```python
from build123d import *

# Parameters (mm, degrees)
BOSS_EXTRUDE1_DEPTH                                = 12.7
F_1_4_20_TAPPED_HOLE1_D                            = 5.1054
F_1_4_20_TAPPED_HOLE1_DEPTH                        = 12.7
F_1_4_20_TAPPED_HOLE2_D                            = 5.1054
F_1_4_20_TAPPED_HOLE2_DEPTH                        = 12.7
LPATTERN1_COUNT                                    = 3
LPATTERN1_PITCH                                    = 12.7
LPATTERN2_COUNT                                    = 3
LPATTERN2_PITCH                                    = 12.7
CSK_FOR_10_FLAT_HEAD_MACHINE_SCREW_100_D           = 5.1054
CSK_FOR_10_FLAT_HEAD_MACHINE_SCREW_100_DEPTH       = 12.7
CSK_FOR_10_FLAT_HEAD_MACHINE_SCREW_100_CSINK_D     = 9.779
CSK_FOR_10_FLAT_HEAD_MACHINE_SCREW_100_CSINK_ANGLE = 100
F_1_8_0_125_DIAMETER_HOLE1_D                       = 3.175
F_1_8_0_125_DIAMETER_HOLE1_DEPTH                   = 12.7
CSK_FOR_10_FLAT_HEAD_MACHINE_SCREW_2_D             = 5.1054
CSK_FOR_10_FLAT_HEAD_MACHINE_SCREW_2_DEPTH         = 12.7
CSK_FOR_10_FLAT_HEAD_MACHINE_SCREW_2_CSINK_D       = 9.779
CSK_FOR_10_FLAT_HEAD_MACHINE_SCREW_2_CSINK_ANGLE   = 100


with BuildPart() as part:
    # Sketch1 → Boss-Extrude1 (new body)
    with BuildSketch(Plane(origin=(0, 0, 0), x_dir=(1, 0, 0), z_dir=(0, 1, 0))):
        Polygon((24.616308072, 0), (53.826308072, 0), (53.826308072, 40.5892), (24.616308072, 40.5892), (24.616308072, 109.3724), (-0.783691928, 109.3724), (-0.783691928, 52.2224), (7.674508072, 52.2224), (8.4582, -11.6332), (-0.783691928, -11.6332), (-0.783691928, -68.7832), (24.616308072, -68.7832), align=None)
    extrude(amount=BOSS_EXTRUDE1_DEPTH)

    # 1/4-20 Tapped Hole1
    with Locations(Plane(origin=(0, 12.7, 0), x_dir=(1, 0, 0), z_dir=(0, 1, 0))):
        with Locations((9.376308072, 99.2124)):
            f_1_4_20_tapped_hole1 = Hole(F_1_4_20_TAPPED_HOLE1_D / 2, depth=F_1_4_20_TAPPED_HOLE1_DEPTH)

    # 1/4-20 Tapped Hole2
    with Locations(Plane(origin=(0, 12.7, 0), x_dir=(1, 0, 0), z_dir=(0, 1, 0))):
        with Locations((9.376308072, -58.6232)):
            f_1_4_20_tapped_hole2 = Hole(F_1_4_20_TAPPED_HOLE2_D / 2, depth=F_1_4_20_TAPPED_HOLE2_DEPTH)

    # LPattern1: 1/4-20 Tapped Hole1 ×3
    with Locations(*[(0, 0, i * LPATTERN1_PITCH) for i in range(1, LPATTERN1_COUNT)]):
        add(f_1_4_20_tapped_hole1, mode=Mode.SUBTRACT)

    # LPattern2: 1/4-20 Tapped Hole2 ×3
    with Locations(*[(0, 0, -i * LPATTERN2_PITCH) for i in range(1, LPATTERN2_COUNT)]):
        add(f_1_4_20_tapped_hole2, mode=Mode.SUBTRACT)

    # CSK for _10 Flat Head Machine Screw _100
    with Locations(Plane(origin=(0, 12.7, 0), x_dir=(1, 0, 0), z_dir=(0, 1, 0))):
        with Locations((35.411308072, 20.2946), (35.411308072, 34.326173542), (35.411308072, 6.960743489)):
            CounterSinkHole(CSK_FOR_10_FLAT_HEAD_MACHINE_SCREW_100_D / 2, CSK_FOR_10_FLAT_HEAD_MACHINE_SCREW_100_CSINK_D / 2, depth=CSK_FOR_10_FLAT_HEAD_MACHINE_SCREW_100_DEPTH, counter_sink_angle=CSK_FOR_10_FLAT_HEAD_MACHINE_SCREW_100_CSINK_ANGLE)

    # 1/8 (0.125) Diameter Hole1
    with Locations(Plane(origin=(0, 12.7, 0), x_dir=(1, 0, 0), z_dir=(0, 1, 0))):
        with Locations((21.441308072, 38.0492), (22.214178029, 2.54), (50.651308072, 3.175), (50.651308072, 37.4142)):
            Hole(F_1_8_0_125_DIAMETER_HOLE1_D / 2, depth=F_1_8_0_125_DIAMETER_HOLE1_DEPTH)

    # CSK for _10 Flat Head Machine Screw  2
    with Locations(Plane(origin=(0, 12.7, 0), x_dir=(1, 0, 0), z_dir=(0, 1, 0))):
        with Locations((47.260541085, 20.2946), (23.544844519, 20.2946)):
            CounterSinkHole(CSK_FOR_10_FLAT_HEAD_MACHINE_SCREW_2_D / 2, CSK_FOR_10_FLAT_HEAD_MACHINE_SCREW_2_CSINK_D / 2, depth=CSK_FOR_10_FLAT_HEAD_MACHINE_SCREW_2_DEPTH, counter_sink_angle=CSK_FOR_10_FLAT_HEAD_MACHINE_SCREW_2_CSINK_ANGLE)


solid = part.part
```
CAD build for the part. Positions are in the model's coordinates, mm. A direction names the side the tool comes from. Round coordinates to 2 decimals unless told otherwise and drop trailing zeros. Use a Markdown table: item, result. Add a question column.
(1) Which spindle directions (+Z, -Z, +X, -X, +Y, -Y) get a long thin tool onto all of the face, cutting with end or side? Do faces 3 (the face through (3, 6, -52.222)), 4 (the face through (39, 6, 0)), 5 (the face through (39, 6, -40.589)). Say none if no direction does.
(2) Drill centre lines: line 1 (Z direction, x = 3.5, y = 2.25); line 2 (X direction, y = 7, z = 20); line 3 (X direction, y = 1.5, z = -88.5). Where is each one in solid material? Low to high.
(3) Pull direction X, two halves, no side cores. Call faces 1 (the face through (22.37, 5.29, -18.03)), 2 (the face through (14, 12.7, -22)): +X half, -X half, draft (parallel to the pull), parting line (faces both ways), or undercut.
(4) Flat gauge pins, fed straight in: pin 1 (1.5 mm diameter, centred on y = 6, z = -54.5, fed in from +X); pin 2 (2.5 mm diameter, centred on x = 22.21, z = -2.54, fed in from -Y); pin 3 (6.5 mm diameter, centred on x = 40.5, y = 4, fed in from +Z); pin 4 (6.5 mm diameter, centred on x = 34, y = 7, fed in from -Z). Where does each tip first touch, or does it go through?
(5) Cut at A-A (y = 4.75). State how many separate pieces and enclosed holes the cut face has, and give its area (3 significant figures).
Geometry says:
| question | item | result |
|---|---|---|
| 1 | face 3 | -X, +Y, -Y |
| 1 | face 4 | +Z, +X, +Y, -Y |
| 1 | face 5 | -Z, +X, +Y, -Y |
| 2 | line 1 | z = -109.37 to -52.22, 11.63 to 68.78 |
| 2 | line 2 | x = -0.78 to 24.62 |
| 2 | line 3 | x = -0.78 to 7.77, 10.98 to 24.62 |
| 3 | face 1 | undercut |
| 3 | face 2 | draft |
| 4 | pin 1 | stops at x = 24.62 |
| 4 | pin 2 | passes through |
| 4 | pin 3 | stops at z = 0 |
| 4 | pin 4 | stops at z = -40.59 |
| 5 | separate pieces | 1 |
| 5 | enclosed holes | 15 |
| 5 | area | 4,890 mm² |
